from build123d import *
from build123d.topology import SkipClean

# Parameters (mm, degrees)
SKETCH1_R            = 7.25
BOSS_EXTRUDE1_DEPTH  = 25
SKETCH2_R            = 2.1
BOSS_EXTRUDE2_DEPTH  = 2.5
SKETCH4_R            = 8.5
BOSS_EXTRUDE3_DEPTH  = 1.5
BOSS_EXTRUDE5_DEPTH  = 12.5
FILLET2_R            = 2
BOSS_EXTRUDE6_START  = 11.25
SKETCH6_R            = 7.25
BOSS_EXTRUDE6_DEPTH  = 11.25
BOSS_EXTRUDE7_START  = 2.5
SKETCH7_R            = 2.1
BOSS_EXTRUDE7_DEPTH  = 2.5
SKETCH8_R            = 2.1
CUT_EXTRUDE1_DEPTH   = 53.5
BOSS_EXTRUDE8_START  = 11.25
SKETCH9_R            = 7.5
SKETCH9_R_2          = 7.25
BOSS_EXTRUDE8_DEPTH  = 11.25
SKETCH10_R           = 7.5
SKETCH10_R_2         = 7.25
BOSS_EXTRUDE9_DEPTH  = 25
SKETCH11_R           = 2.15
CUT_EXTRUDE2_DEPTH   = 50
SKETCH12_R           = 6.607325953
CUT_EXTRUDE3_DEPTH   = 2.5
SKETCH13_R           = 6.756490311
CUT_EXTRUDE4_DEPTH   = 2.5
SKETCH14_W           = 10
SKETCH14_H           = 7.5
SKETCH14_R           = 2.15
BOSS_EXTRUDE10_DEPTH = 2.5
BOSS_EXTRUDE11_START = 2.5
SKETCH15_R           = 2.5
BOSS_EXTRUDE11_DEPTH = 2.5
SKETCH16_R           = 2.5
CUT_EXTRUDE5_DEPTH   = 61.5


with BuildPart() as part:
    # Sketch1 → Boss-Extrude1 (new body)
    with BuildSketch(Plane(origin=(0, 0, 0), x_dir=(1, 0, 0), z_dir=(0, 1, 0))):
        with Locations(Location((0, 0, 0), (0, 0, 270))):
            Circle(SKETCH1_R)
    extrude(amount=BOSS_EXTRUDE1_DEPTH)

    # Sketch2 → Boss-Extrude2 (add)
    with BuildSketch(Plane(origin=(0, 25, 0), x_dir=(1, 0, 0), z_dir=(0, 1, 0))):
        with BuildLine():
            Line((-4.9, -3.65), (4.9, -3.65))
            ThreePointArc((4.9, -3.65), (5.781186897, 0), (4.9, 3.65))
            Line((4.9, 3.65), (-4.9, 3.65))
            ThreePointArc((-4.9, 3.65), (-5.781186897, 0), (-4.9, -3.65))
        make_face()
        with Locations(Location((0, 0, 0), (0, 0, 270))):
            Circle(SKETCH2_R, mode=Mode.SUBTRACT)
    extrude(amount=BOSS_EXTRUDE2_DEPTH)

    # Sketch4 → Boss-Extrude3 (add)
    with BuildSketch(Plane(origin=(0, 0, 0), x_dir=(-1, 0, 0), z_dir=(0, -1, 0))):
        with Locations(Location((0, 0, 0), (0, 0, 90))):
            Circle(SKETCH4_R)
    extrude(amount=BOSS_EXTRUDE3_DEPTH)

    # Sketch5 → Boss-Extrude5 (add)
    with SkipClean():  # the faces are left unmerged after this step: merging them gives an invalid solid
        with BuildSketch(Plane(origin=(0, 0, 0), x_dir=(1, 0, 0), z_dir=(0, 1, 0))):
            with BuildLine():
                Line((-2.25, 8.196798155), (-2.25, 6.892024376))
                ThreePointArc((-2.25, 6.892024376), (0, 7.25), (2.25, 6.892024376))
                Line((2.25, 6.892024376), (2.25, 8.196798155))
                ThreePointArc((2.25, 8.196798155), (0, 8.5), (-2.25, 8.196798155))
            make_face()
            with BuildLine():
                Line((6.892024376, 2.25), (8.196798155, 2.25))
                ThreePointArc((8.196798155, 2.25), (8.5, 0), (8.196798155, -2.25))
                Line((8.196798155, -2.25), (6.892024376, -2.25))
                ThreePointArc((6.892024376, -2.25), (7.25, 0), (6.892024376, 2.25))
            make_face()
            with BuildLine():
                Line((2.25, -8.196798155), (2.25, -6.892024376))
                ThreePointArc((2.25, -6.892024376), (0, -7.25), (-2.25, -6.892024376))
                Line((-2.25, -6.892024376), (-2.25, -8.196798155))
                ThreePointArc((-2.25, -8.196798155), (0, -8.5), (2.25, -8.196798155))
            make_face()
            with BuildLine():
                Line((-6.892024376, -2.25), (-8.196798155, -2.25))
                ThreePointArc((-8.196798155, -2.25), (-8.5, 0), (-8.196798155, 2.25))
                Line((-8.196798155, 2.25), (-6.892024376, 2.25))
                ThreePointArc((-6.892024376, 2.25), (-7.25, 0), (-6.892024376, -2.25))
            make_face()
        extrude(amount=BOSS_EXTRUDE5_DEPTH)

    # Fillet2
    # the kernel refuses this fillet: 2 mm, written as the material it takes off along each edge
    with BuildSketch(Plane(origin=(0, 12.5, 0), x_dir=(-0.6871531367836845, 0, 0.72651260595281), z_dir=(0.72651260595281, 0, 0.6871531367836845))) as fillet2_piece_1:
        with BuildLine():
            CenterArc((6.5, 1.854049622), FILLET2_R, 292.024312837, 67.975687163)
            Line((7.25, 0), (7.265, -0.037080992))
            ThreePointArc((7.265, -0.037080992), (7.875, -0.04), (8.5, -0.04))
            Line((8.5, -0.04), (8.54, 0))
            Line((8.54, 0), (8.54, 1.854049622))
            Line((8.54, 1.854049622), (8.5, 1.854049622))
        make_face()
    revolve(axis=Axis((0, 12.5, 0), (0, -1, 0)), revolution_arc=93.189649372, mode=Mode.SUBTRACT)
    with BuildSketch(Plane(origin=(0, 12.5, 0), x_dir=(0.7265126059528094, 0, -0.687153136783685), z_dir=(0.687153136783685, 0, 0.7265126059528094))) as fillet2_piece_2:
        with BuildLine():
            CenterArc((6.5, -1.854049622), FILLET2_R, 0, 67.975687163)
            Line((7.25, 0), (7.265, 0.037080992))
            ThreePointArc((7.265, 0.037080992), (7.875, 0.04), (8.5, 0.04))
            Line((8.5, 0.04), (8.54, 0))
            Line((8.54, 0), (8.54, -1.854049622))
            Line((8.54, -1.854049622), (8.5, -1.854049622))
        make_face()
    revolve(axis=Axis((0, 12.5, 0), (0, 1, 0)), revolution_arc=93.189649372, mode=Mode.SUBTRACT)
    with BuildSketch(Plane(origin=(0, 12.5, 0), x_dir=(0.687153136783685, 0, -0.7265126059528094), z_dir=(-0.7265126059528094, 0, -0.687153136783685))) as fillet2_piece_3:
        with BuildLine():
            CenterArc((6.5, 1.854049622), FILLET2_R, 292.024312837, 67.975687163)
            Line((7.25, 0), (7.265, -0.037080992))
            ThreePointArc((7.265, -0.037080992), (7.875, -0.04), (8.5, -0.04))
            Line((8.5, -0.04), (8.54, 0))
            Line((8.54, 0), (8.54, 1.854049622))
            Line((8.54, 1.854049622), (8.5, 1.854049622))
        make_face()
    revolve(axis=Axis((0, 12.5, 0), (0, -1, 0)), revolution_arc=93.189649372, mode=Mode.SUBTRACT)
    with BuildSketch(Plane(origin=(0, 12.5, 0), x_dir=(-0.7265126059528072, 0, 0.6871531367836876), z_dir=(-0.6871531367836876, 0, -0.7265126059528072))) as fillet2_piece_4:
        with BuildLine():
            CenterArc((6.5, -1.854049622), FILLET2_R, 0, 67.975687163)
            Line((7.25, 0), (7.265, 0.037080992))
            ThreePointArc((7.265, 0.037080992), (7.875, 0.04), (8.5, 0.04))
            Line((8.5, 0.04), (8.54, 0))
            Line((8.54, 0), (8.54, -1.854049622))
            Line((8.54, -1.854049622), (8.5, -1.854049622))
        make_face()
    revolve(axis=Axis((0, 12.5, 0), (0, 1, 0)), revolution_arc=93.189649372, mode=Mode.SUBTRACT)

    # Sketch6 → Boss-Extrude6 (add)
    with BuildSketch(Plane(origin=(0, -1.5, 0), x_dir=(-1, 0, 0), z_dir=(0, -1, 0)).offset(BOSS_EXTRUDE6_START)):
        with Locations(Location((0, 0, 0), (0, 0, 108.080012624))):
            Circle(SKETCH6_R)
    extrude(amount=-BOSS_EXTRUDE6_DEPTH)

    # Sketch7 → Boss-Extrude7 (add)
    with BuildSketch(Plane(origin=(0, -12.75, 0), x_dir=(-1, 0, 0), z_dir=(0, -1, 0)).offset(BOSS_EXTRUDE7_START)):
        with BuildLine():
            Line((4.9, 3.65), (-4.9, 3.65))
            ThreePointArc((-4.9, 3.65), (-5.781186897, 0), (-4.9, -3.65))
            Line((-4.9, -3.65), (4.9, -3.65))
            ThreePointArc((4.9, -3.65), (5.781186897, 0), (4.9, 3.65))
        make_face()
        with Locations(Location((0, 0, 0), (0, 0, 270))):
            Circle(SKETCH7_R, mode=Mode.SUBTRACT)
    extrude(amount=-BOSS_EXTRUDE7_DEPTH)

    # Sketch8 → Cut-Extrude1 (cut)
    with BuildSketch(Plane(origin=(0, -12.75, 0), x_dir=(-1, 0, 0), z_dir=(0, -1, 0))):
        with Locations(Location((0, 0, 0), (0, 0, 90))):
            Circle(SKETCH8_R)
    extrude(amount=-CUT_EXTRUDE1_DEPTH, mode=Mode.SUBTRACT)

    # Sketch9 → Boss-Extrude8 (add)
    with BuildSketch(Plane.XZ.offset(1.5).offset(BOSS_EXTRUDE8_START)):
        with Locations(Location((0, 0, 0), (0, 0, 270))):
            Circle(SKETCH9_R)
        with Locations(Location((0, 0, 0), (0, 0, 288.080012624))):
            Circle(SKETCH9_R_2, mode=Mode.SUBTRACT)
    extrude(amount=-BOSS_EXTRUDE8_DEPTH)

    # Sketch10 → Boss-Extrude9 (add)
    with BuildSketch(Plane(origin=(0, 0, 0), x_dir=(1, 0, 0), z_dir=(0, 1, 0))):
        with Locations(Location((0, 0, 0), (0, 0, 90))):
            Circle(SKETCH10_R)
        Circle(SKETCH10_R_2, mode=Mode.SUBTRACT)
    extrude(amount=BOSS_EXTRUDE9_DEPTH)

    # Sketch11 → Cut-Extrude2 (cut)
    with BuildSketch(Plane(origin=(0, 27.5, 0), x_dir=(1, 0, 0), z_dir=(0, 1, 0))):
        with Locations(Location((0, 0, 0), (0, 0, 270))):
            Circle(SKETCH11_R)
    extrude(amount=-CUT_EXTRUDE2_DEPTH, mode=Mode.SUBTRACT)

    # Sketch12 → Cut-Extrude3 (cut)
    with BuildSketch(Plane(origin=(0, -15.25, 0), x_dir=(-1, 0, 0), z_dir=(0, -1, 0))):
        Circle(SKETCH12_R)
    extrude(amount=-CUT_EXTRUDE3_DEPTH, mode=Mode.SUBTRACT)

    # Sketch13 → Cut-Extrude4 (cut)
    with BuildSketch(Plane(origin=(0, 27.5, 0), x_dir=(1, 0, 0), z_dir=(0, 1, 0))):
        Circle(SKETCH13_R)
    extrude(amount=-CUT_EXTRUDE4_DEPTH, mode=Mode.SUBTRACT)

    # Sketch14 → Boss-Extrude10 (add)
    # profile 1 of 3: a face of its own
    with BuildSketch(Plane(origin=(0, -12.75, 0), x_dir=(-1, 0, 0), z_dir=(0, -1, 0))):
        Rectangle(SKETCH14_W, SKETCH14_H)
        with Locations(Location((0, 0, 0), (0, 0, 270))):
            Circle(SKETCH14_R, mode=Mode.SUBTRACT)
    # profile 2 of 3: a face of its own
    with BuildSketch(Plane(origin=(0, -12.75, 0), x_dir=(-1, 0, 0), z_dir=(0, -1, 0))):
        with BuildLine():
            Line((5, 3.75), (5, -3.75))
            ThreePointArc((5, -3.75), (5.933352987, 0), (5, 3.75))
        make_face()
    # profile 3 of 3: a face of its own
    with BuildSketch(Plane(origin=(0, -12.75, 0), x_dir=(-1, 0, 0), z_dir=(0, -1, 0))):
        with BuildLine():
            ThreePointArc((-5, -3.75), (-5.933352987, 0), (-5, 3.75))
            Line((-5, 3.75), (-5, -3.75))
        make_face()
    extrude(amount=BOSS_EXTRUDE10_DEPTH)

    # Sketch15 → Boss-Extrude11 (add)
    with BuildSketch(Plane(origin=(0, 25, 0), x_dir=(1, 0, 0), z_dir=(0, 1, 0)).offset(BOSS_EXTRUDE11_START)):
        with BuildLine():
            Line((-5, -3.75), (5, -3.75))
            ThreePointArc((5, -3.75), (5.933352987, 0), (5, 3.75))
            Line((5, 3.75), (-5, 3.75))
            ThreePointArc((-5, 3.75), (-5.933352987, 0), (-5, -3.75))
        make_face()
        with Locations(Location((0, 0, 0), (0, 0, 270))):
            Circle(SKETCH15_R, mode=Mode.SUBTRACT)
    extrude(amount=-BOSS_EXTRUDE11_DEPTH)

    # Sketch16 → Cut-Extrude5 (cut)
    with BuildSketch(Plane(origin=(0, 25, 0), x_dir=(1, 0, 0), z_dir=(0, 1, 0))):
        with Locations(Location((0, 0, 0), (0, 0, 90))):
            Circle(SKETCH16_R)
    extrude(amount=-CUT_EXTRUDE5_DEPTH, mode=Mode.SUBTRACT)


solid = part.part
Check sheet for the modelled part. Datum: model origin and axes. Units: mm. A direction names the side the tool comes from. Coordinates: 2 decimals unless noted, no trailing zeros. Loops run counter-clockwise (first coordinate to the right, second up) from the corner with the lowest first, then second, coordinate; pieces in that order, holes last. Notation, with made-up numbers: (38.25, 51) -> (71.25, 51) arc R6 ccw to (71.25, 55) -> close; hole circle Ø9 at (-25, 8). An arc over 180 degrees is marked (long way). Write item = value, one per line. Start each with the question number.
1. Section check A-A on y = 10. Record the cut outline in (x, z), then the cut area to 3 significant figures.
2. Section check C-C on z = 0. Record the cut outline in (x, y).
3. Material ranges on line 1 (X direction, y = 26.7, z = 0); line 2 (Y direction, x = 6.5, z = -3); line 3 (X direction, y = 3, z = -0.5), recorded low to high.
4. Depth check by flat-ended pin: P1, Ø6.5, axis at x = -4, z = 4, coming from the +Y side; P2, Ø2, axis at y = 17.5, z = 3, coming from the +X side; P3, Ø0.8, axis at x = 1, y = 26.5, coming from the +Z side; P4, Ø2, axis at x = 0, y = -14.5, coming from the -Z side. Enter the tip coordinate at first touch or a pass-through.
5. Section check D-D on x = -3.5. Record the cut outline in (y, z), then the cut area to 3 significant figures.
6. Tool access check on faces 1 (the flat face through (8, 6, 2.25)), 2 (the flat face through (-5.43, 0, -5.43)), 3 (the cylindrical face through (2.87, 12.32, -6.93)), 4 (the cylindrical face through (-5.933, 26.268, -0.055)), 5 (the flat face through (8, 6, -2.25)). Record the directions out of +Z, -Z, +X, -X, +Y, -Y that give a thin tool (end or side, any length) a straight path to the whole face; none if there is none.
7. Section check B-B on x = 0. Record the cut outline in (y, z), then the cut area to 3 significant figures.
Responses:
q1.outline = (-8.2, -2.25) -> (-7.15, -2.25) arc R7.5 ccw to (-2.25, -7.15) -> (-2.25, -8.2) arc R8.5 ccw to (2.25, -8.2) -> (2.25, -7.15) arc R7.5 ccw to (7.15, -2.25) -> (8.2, -2.25) arc R8.5 ccw to (8.2, 2.25) -> (7.15, 2.25) arc R7.5 ccw to (2.25, 7.15) -> (2.25, 8.2) arc R8.5 ccw to (-2.25, 8.2) -> (-2.25, 7.15) arc R7.5 ccw to (-7.15, 2.25) -> (-8.2, 2.25) arc R8.5 ccw to start; hole circle Ø5 at (0, 0)
q1.area = 175 mm2
q2.outline = (-8.5, -1.5) -> (-7.5, -1.5) -> (-7.5, -12.75) -> (-5.93, -12.75) -> (-5.93, -15.25) -> (-2.5, -15.25) -> (-2.5, 27.5) -> (-5.93, 27.5) -> (-5.93, 25) -> (-7.5, 25) -> (-7.5, 12.38) arc R2 ccw to (-8.5, 10.65) -> close; (2.5, -15.25) -> (5.93, -15.25) -> (5.93, -12.75) -> (7.5, -12.75) -> (7.5, -1.5) -> (8.5, -1.5) -> (8.5, 10.65) arc R2 ccw to (7.5, 12.38) -> (7.5, 25) -> (5.93, 25) -> (5.93, 27.5) -> (2.5, 27.5) -> close
q3.line_1 = -5.93 to -2.5, 2.5 to 5.93
q3.line_2 = -12.75 to 25
q3.line_3 = -8.49 to -2.45, 2.45 to 8.49
q4.P1 = 27.5
q4.P2 = 7.23
q4.P3 = 3.75
q4.P4 = -3.75
q5.outline = (-15.25, -3.75) -> (-12.75, -3.75) -> (-12.75, -6.63) -> (-1.5, -6.63) -> (-1.5, -7.75) -> (0, -7.75) -> (0, -6.63) -> (25, -6.63) -> (25, -3.75) -> (27.5, -3.75) -> (27.5, 3.75) -> (25, 3.75) -> (25, 6.63) -> (0, 6.63) -> (0, 7.75) -> (-1.5, 7.75) -> (-1.5, 6.63) -> (-12.75, 6.63) -> (-12.75, 3.75) -> (-15.25, 3.75) -> close
q5.area = 542 mm2
q6.face_1 = +Z, +X, +Y
q6.face_2 = -Z, -X, +Y
q6.face_3 = +Y
q6.face_4 = -X, +Y
q6.face_5 = -Z, +X, +Y
q7.outline = (-15.25, -3.75) -> (-12.75, -3.75) -> (-12.75, -7.5) -> (-1.5, -7.5) -> (-1.5, -8.5) -> (10.65, -8.5) arc R2 ccw to (12.38, -7.5) -> (25, -7.5) -> (25, -3.75) -> (27.5, -3.75) -> (27.5, -2.5) -> (-15.25, -2.5) -> close; (-15.25, 2.5) -> (27.5, 2.5) -> (27.5, 3.75) -> (25, 3.75) -> (25, 7.5) -> (12.38, 7.5) arc R2 ccw to (10.65, 8.5) -> (-1.5, 8.5) -> (-1.5, 7.5) -> (-12.75, 7.5) -> (-12.75, 3.75) -> (-15.25, 3.75) -> close
q7.area = 417 mm2
